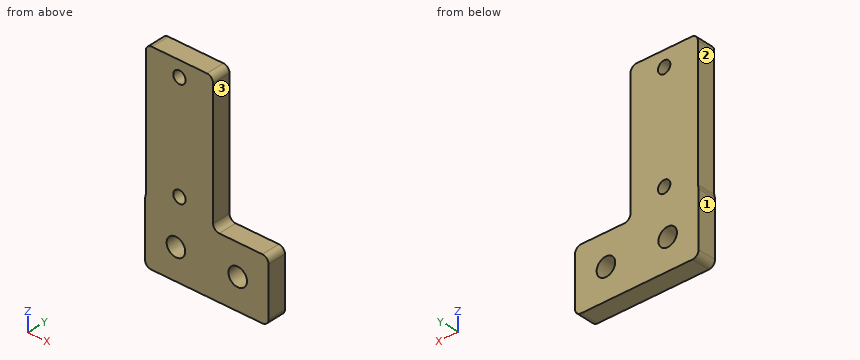
```python
from build123d import *

# Parameters (mm, degrees)
SKETCH1_R           = 1.5
SKETCH1_R_2         = 1
BOSS_EXTRUDE1_DEPTH = 3
FILLET2_R           = 1
FILLET5_R           = 1
FILLET6_R           = 1


with BuildPart() as part:
    # Sketch1 → Boss-Extrude1 (new body)
    with BuildSketch(Plane(origin=(0, 0, 0), x_dir=(1, 0, 0), z_dir=(0, 1, 0))):
        Polygon((11.02, 0), (20, 0), (20, 10), (0, 10), (0, 0), (0.12, 0), (0.12, -22.3), (11.02, -22.3), align=None)
        with Locations(Location((5, 5, 0), (0, 0, 270))):
            Circle(SKETCH1_R, mode=Mode.SUBTRACT)
        with Locations(Location((15, 5, 0), (0, 0, 270))):
            Circle(SKETCH1_R, mode=Mode.SUBTRACT)
        with Locations(Location((5.57, -2.5, 0), (0, 0, 270))):
            Circle(SKETCH1_R_2, mode=Mode.SUBTRACT)
        with Locations(Location((5.57, -19.8, 0), (0, 0, 270))):
            Circle(SKETCH1_R_2, mode=Mode.SUBTRACT)
    extrude(amount=BOSS_EXTRUDE1_DEPTH)

    # Fillet2
    fillet2_edges = [part.edges().sort_by_distance(p)[0] for p in [
        (11.02, 1.5, 22.3),
        (0.12, 1.5, 22.3),
        (0, 1.5, -10),
        (20, 1.5, -10),
        (20, 1.5, 0),
        (11.02, 1.5, 0),
    ]]
    fillet(fillet2_edges, radius=FILLET2_R)

    # Fillet5
    # the kernel refuses this fillet: 1 mm, written as the material it adds along each edge
    with BuildSketch(Plane(origin=(0.12, 0, 0), x_dir=(0, 0, 1), z_dir=(0, 1, 0))) as fillet5_piece_1:
        with BuildLine():
            CenterArc((0.474973683, -1), FILLET5_R, 90, 28.357636576)
            Line((0, -0.12), (-0.009499474, -0.1024))
            ThreePointArc((-0.009499474, -0.1024), (-0.02, -0.06), (-0.02, 0))
            Line((-0.02, 0), (0, 0.02))
            Line((0, 0.02), (0.474973683, 0.02))
            Line((0.474973683, 0.02), (0.474973683, 0))
        make_face()
    extrude(amount=3)

    # Fillet6
    fillet6_edges = [part.edges().sort_by_distance(p)[0] for p in [
        (0, 1.5, 0),
    ]]
    fillet(fillet6_edges, radius=FILLET6_R)


solid = part.part
```
Geometry: final body of the model. Coordinates: model frame, mm. Face numbers are marked on the shaded views. A direction names the side the tool comes from. Coordinates: 2 decimals unless noted, no trailing zeros. Order: outer loops, then holes, each group sorted by start corner. A loop starts at its lowest first (then second) coordinate and runs counter-clockwise, first axis right, second up. Notation, with made-up numbers: M -2.5,10 L 16.5,10 A4 ccw 16.5,16 Z; hole C 73.25,31 d10. An arc over 180 degrees is marked long. Answer in a Markdown table with one row per item. Add a question column.
Q1. Line query: L1, parallel to X at y = 2.25, z = -5; L2, parallel to X at y = 0.8, z = 2.5; L3, parallel to X at y = 1.7, z = -4.5. Output: solid intervals per line, ascending.
Q2. Reachability of the marked faces 1, 2 and 3 from +Z, -Z, +X, -X, +Y, -Y: full face, straight path, thin tool, end or side. Return the list, or none.
Q3. Section query B-B on z = 2.5. Return the cut outline in (x, y).
Q4. Contact query for flat-ended pins moving along their axis: P1, Ø2.5, axis at x = 5, z = -5, coming from the -Y side; P2, Ø1.5, axis at y = 2, z = 13.5, coming from the +X side. Output: stop coordinate, or through.
Q5. Section query A-A on x = 15. Return the cut outline in (y, z), and give its area (3 significant figures).
Q6. Section query D-D on x = 5. Return the cut outline in (y, z).
Q7. Section query C-C on y = 1.15. Return the cut outline in (x, z).
Completed:
| question | item | result |
|---|---|---|
| 1 | L1 | x = 0 to 3.5, 6.5 to 13.5, 16.5 to 20 |
| 1 | L2 | x = 0.12 to 4.57, 6.57 to 11.02 |
| 1 | L3 | x = 0 to 3.59, 6.41 to 13.59, 16.41 to 20 |
| 2 | face 1 | +Z, -Z, -X, +Y, -Y |
| 2 | face 2 | +Z, -X, +Y, -Y |
| 2 | face 3 | +Z, +X, +Y, -Y |
| 3 | outline | M 0.12,0 L 4.57,0 L 4.57,3 L 0.12,3 Z; M 6.57,0 L 11.02,0 L 11.02,3 L 6.57,3 Z |
| 4 | P1 | passes through |
| 4 | P2 | stops at x = 11.02 |
| 5 | outline | M 0,-10 L 3,-10 L 3,-6.5 L 0,-6.5 Z; M 0,-3.5 L 3,-3.5 L 3,0 L 0,0 Z |
| 5 | area | 21.0 mm2 |
| 6 | outline | M 0,-10 L 3,-10 L 3,-6.5 L 0,-6.5 Z; M 0,-3.5 L 3,-3.5 L 3,1.68 L 0,1.68 Z; M 0,3.32 L 3,3.32 L 3,18.98 L 0,18.98 Z; M 0,20.62 L 3,20.62 L 3,22.3 L 0,22.3 Z |
| 7 | outline | M 0,-9 A1 ccw 1,-10 L 19,-10 A1 ccw 20,-9 L 20,-1 A1 ccw 19,0 L 12.02,0 A1 cw 11.02,1 L 11.02,21.3 A1 ccw 10.02,22.3 L 1.12,22.3 A1 ccw 0.12,21.3 L 0.12,0.47 A1 cw 0.06,0.13 A1 ccw 0,-0.21 Z; hole C 5,-5 d3; hole C 5.57,2.5 d2; hole C 5.57,19.8 d2; hole C 15,-5 d3 |
